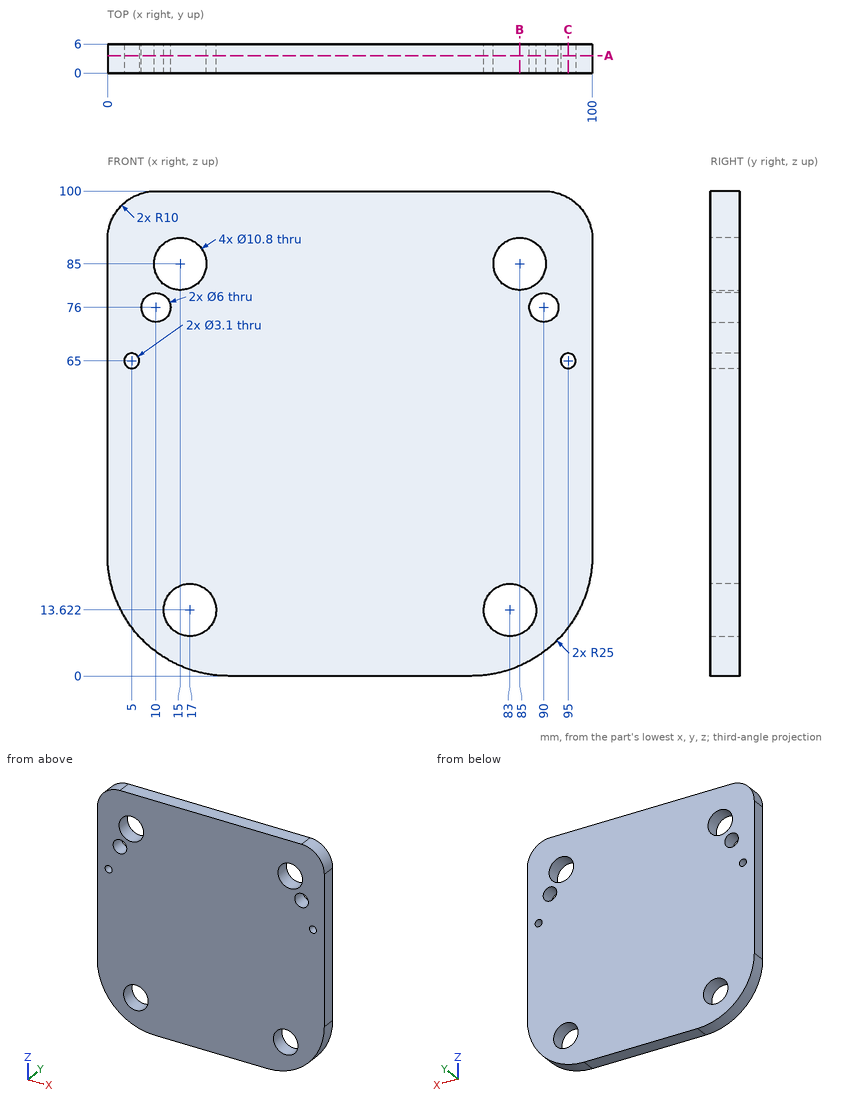
Verification items for this drawing (mm, ordinates from the low corner). Give positions to 0.01 mm unless a question says otherwise; leave off trailing zeros. Loops run counter-clockwise (first coordinate to the right, second up) from the corner with the lowest first, then second, coordinate; pieces in that order, holes last. Notation, with made-up numbers: M 38,-31 L 82,-31 A17 ccw 82,-4 Z; hole C -16,39.5 d11. An arc over 180 degrees is marked long. Write each question's results on one line, items separated by ' | '.
1) Thickness scan on line 1 (X direction, y = 2.15, z = 65); line 2 (Z direction, x = 12, y = 0.85) (1 decimal); line 3 (Z direction, x = 89, y = 4.7). Record the ranges inside material, lowest first.
Answers follow:
line 1: 0 to 3.45, 6.55 to 93.45, 96.55 to 100 | line 2: 3.6 to 11.6, 15.7 to 73.8, 78.2 to 80.5, 89.5 to 100 | line 3: 4.29 to 73.17, 78.83 to 81.37, 88.63 to 100
2) Section check C-C, the plane x = 95. Record the boundary of the cut face in (y, z).
Answers follow:
outline: M 0,10 L 6,10 L 6,63.45 L 0,63.45 Z; M 0,66.55 L 6,66.55 L 6,98.66 L 0,98.66 Z
3) Section check B-B, the plane x = 85. Record the boundary of the cut face in (y, z) (1 decimal).
Answers follow:
outline: M 0,2.1 L 6,2.1 L 6,8.6 L 0,8.6 Z; M 0,18.6 L 6,18.6 L 6,79.6 L 0,79.6 Z; M 0,90.4 L 6,90.4 L 6,100 L 0,100 Z
4) Section check A-A, the plane y = 3.6. Count the separate pieces of the cut face and the enclosed holes in it, plus the area to 3 significant figures.
Answers follow:
separate pieces: 1 | enclosed holes: 8 | area: 9,250 mm2
5) Gauge pin test, flat end, axial feed: pin 1 (1 mm diameter, centred on x = 20.5, y = 2.5, fed in from -Z). Record the tip position at first contact, or that the pin passes through.
Answers follow:
pin 1: z = 0.32
